Job drawing, mm, ordinate dimensions from the low corner. One solid piece. Coordinates: 2 decimals unless noted, no trailing zeros. Loops run counter-clockwise (first coordinate to the right, second up) from the corner with the lowest first, then second, coordinate; pieces in that order, holes last. Notation, with made-up numbers: M 58,49.5 L 67,49.5 A28 cw 67,75.5 Z; hole C 69.25,42.25 d5. An arc over 180 degrees is marked long. Answer as a JSON object with one key per item and string values. Group by question number.
1. Drill centre lines: L1, parallel to Y at x = 19.05, z = 3.75; L2, parallel to X at y = 20, z = 4; L3, parallel to X at y = 135, z = 6.25 (1 decimal). Where is each one in solid material? Low to high.
2. Saw through at A-A on y = 57.15. Write the cut outline in (x, z), then the cut area to 3 significant figures.
3. Saw through at C-C on z = 1. Write the cut outline in (x, y).
4. Saw through at D-D on y = 19.05. Write the cut outline in (x, z), then the cut area to 3 significant figures.
5. Drop flat-ended pins along their axis: pin 1 Ø9.5 at (x, y) = (19.05, 95.25) entering from -Z; pin 2 Ø8 at (x, y) = (100, 101.5) entering from -Z. Give the stop position or say it passes through.
6. Saw through at B-B on x = 95.25. Write the cut outline in (y, z), then the cut area to 3 significant figures.
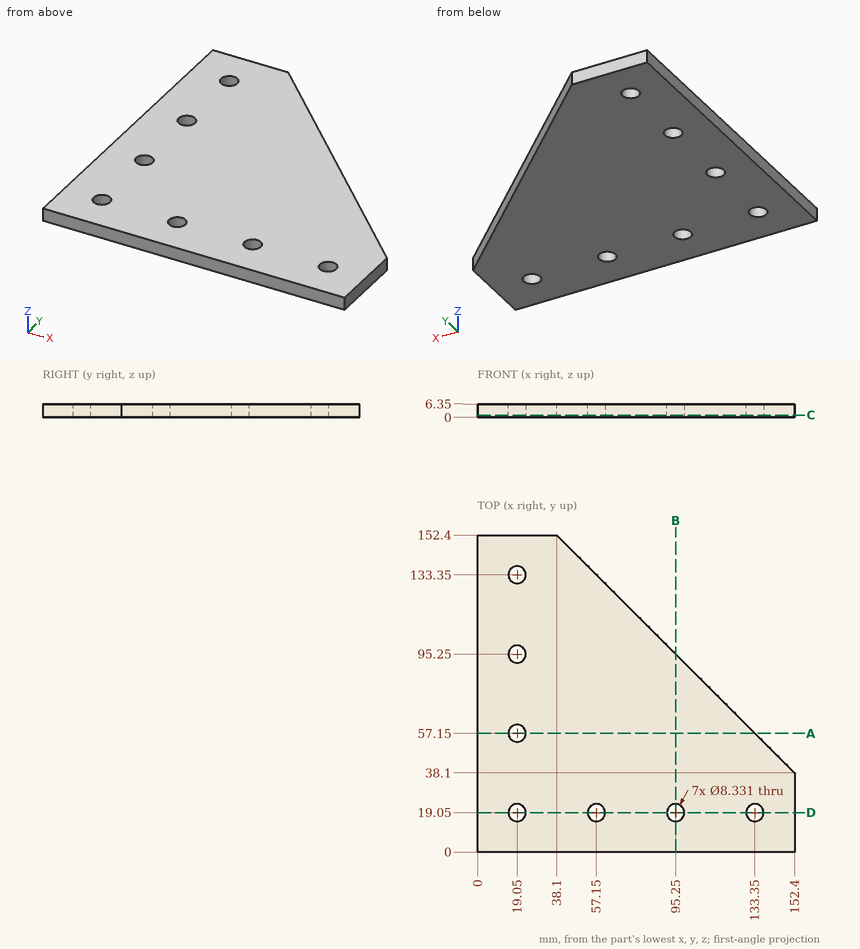
Outcome:
{
 "1": {"L1": "y = 0 to 14.88, 23.22 to 52.98, 61.32 to 91.08, 99.42 to 129.18, 137.52 to 152.4", "L2": "x = 0 to 14.99, 23.11 to 53.09, 61.21 to 91.19, 99.31 to 129.29, 137.41 to 152.4", "L3": "x = 0 to 15.2, 22.9 to 55.5"},
 "2": {"outline": "M 0,0 L 14.88,0 L 14.88,6.35 L 0,6.35 Z; M 23.22,0 L 133.35,0 L 133.35,6.35 L 23.22,6.35 Z", "area": "794 mm²"},
 "3": {"outline": "M 0,0 L 152.4,0 L 152.4,38.1 L 38.1,152.4 L 0,152.4 Z; hole C 19.05,19.05 d8.33; hole C 19.05,57.15 d8.33; hole C 19.05,95.25 d8.33; hole C 19.05,133.35 d8.33; hole C 57.15,19.05 d8.33; hole C 95.25,19.05 d8.33; hole C 133.35,19.05 d8.33"},
 "4": {"outline": "M 0,0 L 14.88,0 L 14.88,6.35 L 0,6.35 Z; M 23.22,0 L 52.98,0 L 52.98,6.35 L 23.22,6.35 Z; M 61.32,0 L 91.08,0 L 91.08,6.35 L 61.32,6.35 Z; M 99.42,0 L 129.18,0 L 129.18,6.35 L 99.42,6.35 Z; M 137.52,0 L 152.4,0 L 152.4,6.35 L 137.52,6.35 Z", "area": "756 mm²"},
 "5": {"pin 1": "stops at z = 0", "pin 2": "passes through"},
 "6": {"outline": "M 0,0 L 14.88,0 L 14.88,6.35 L 0,6.35 Z; M 23.22,0 L 95.25,0 L 95.25,6.35 L 23.22,6.35 Z", "area": "552 mm²"}
}
